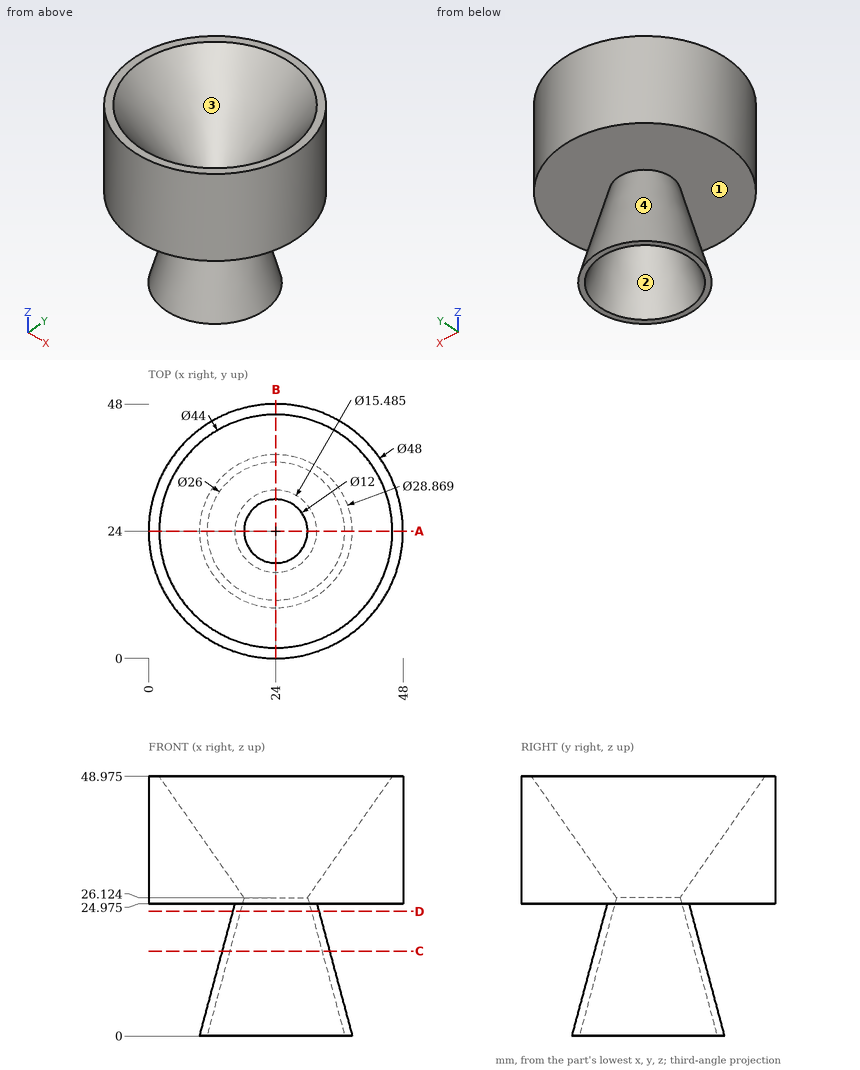
Source: three-view drawing plus pictorial views. Frame: mm from the lowest corner of the part. Give positions to 0.01 mm unless a question says otherwise; leave off trailing zeros. Loops run counter-clockwise (first coordinate to the right, second up) from the corner with the lowest first, then second, coordinate; pieces in that order, holes last. Notation, with made-up numbers: (14.25, 34) -> (71.25, 34) arc R23 cw to (71.25, 48) -> close; hole circle Ø2 at (26.5, 86). An arc over 180 degrees is marked (long way). Put each result on its own line as item: value. Start each with the question number.
1) Cut plane D-D (z = 23.5). Return loops of the section in (x, y) (1 decimal).
2) Material intervals for probe 1 along X at (y, z) = (29, 42) (1 decimal); probe 2 along X at (y, z) = (16, 12) (1 decimal); probe 3 along Y at (x, z) = (22.5, 14), sorted ascending.
3) Cut plane A-A (y = 24). Return loops of the section in (x, z) (1 decimal).
4) Cut plane C-C (z = 16). Return loops of the section in (x, y) (1 decimal).
5) Draft query along X for the marked faces 1, 2, 3 and 4. Return one class per face: released by +X, released by -X, zero draft, split by the parting line, or undercut.
6) Contact query for flat-ended pins moving along their axis: P1, Ø3, axis at y = 22.5, z = 24.5, coming from the -X side; P2, Ø4, axis at y = 37, z = 30.5, coming from the -X side; P3, Ø1.5, axis at x = 37, y = 14, coming from the +Z side; P4, Ø3, axis at x = 34, y = 36, coming from the -Z side. Output: stop coordinate, or through.
Results are:
1. outline: circle Ø16.3 at (24, 24); hole circle Ø13.4 at (24, 24)
2. probe 1: x = 0.5 to 7.6, 40.4 to 47.5
2. probe 2: x = 16.1 to 18.4, 29.6 to 31.9
2. probe 3: y = 13.42 to 14.87, 33.13 to 34.58
3. outline: (0, 25) -> (16.3, 25) -> (9.6, 0) -> (11, 0) -> (18, 26.1) -> (2, 49) -> (0, 49) -> close; (30, 26.1) -> (37, 0) -> (38.4, 0) -> (31.7, 25) -> (48, 25) -> (48, 49) -> (46, 49) -> close
4. outline: circle Ø20.3 at (24, 24); hole circle Ø17.4 at (24, 24)
5. face 1: zero draft
5. face 2: undercut
5. face 3: undercut
5. face 4: split by the parting line
6. P1: stops at x = 0
6. P2: stops at x = 2.67
6. P3: stops at z = 42.05
6. P4: stops at z = 0
